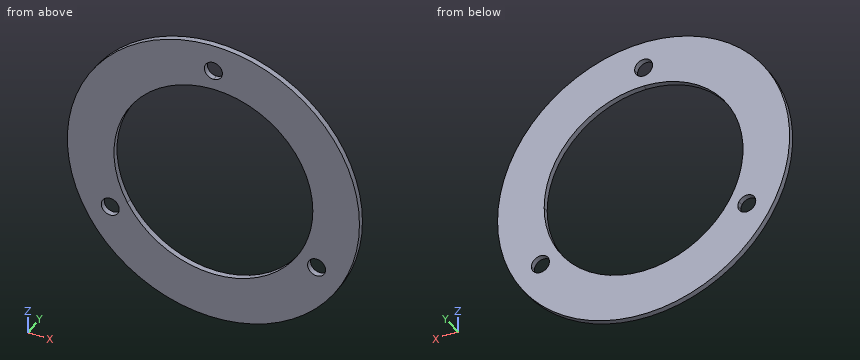
from build123d import *

# Parameters (mm, degrees)
F0_R     = 50.75
F1_DEPTH = 2


with BuildPart() as f1:
    # F0 (on Front) → F1 (new body)
    with BuildSketch(Plane.XZ):
        Circle(F0_R)
        with BuildLine():
            ThreePointArc((-32.725, -20.698007), (-38.868518, -21.506817), (-33.143671, -19.135507))
            ThreePointArc((-33.143671, -19.135507), (-32.831482, -19.889198), (-32.725, -20.698007))
        make_face(mode=Mode.SUBTRACT)
        with BuildLine():
            ThreePointArc((38.975, -20.698007), (35.04119, -23.716525), (33.143671, -19.135507))
            ThreePointArc((33.143671, -19.135507), (36.65881, -17.679489), (38.975, -20.698007))
        make_face(mode=Mode.SUBTRACT)
        with BuildLine():
            ThreePointArc((-29.921178, -17.275), (-29.921178, 17.275), (0, 34.55))
            ThreePointArc((0, 34.55), (24.430539, 24.430539), (34.55, 0))
            ThreePointArc((34.55, 0), (33.372737, -8.942198), (29.921178, -17.275))
            ThreePointArc((29.921178, -17.275), (0, -34.55), (-29.921178, -17.275))
        make_face(mode=Mode.SUBTRACT)
        with BuildLine():
            ThreePointArc((0, 38.271014), (-2.209709, 43.605723), (3.125, 41.396014))
            ThreePointArc((3.125, 41.396014), (2.209709, 39.186306), (0, 38.271014))
        make_face(mode=Mode.SUBTRACT)
    extrude(amount=F1_DEPTH)


solid = f1.part
The listing builds one solid part. Answer for the finished solid, in the listing's coordinates (mm). Give positions to 0.01 mm unless a question says otherwise; leave off trailing zeros. Write each loop counter-clockwise with the first axis right and the second up, starting at its lowest first coordinate (ties: lowest second). Pieces come first, ordered by that corner, then holes. Notation, with made-up numbers: (-25, -13.5) - (-1, -13.5) arc R9 ccw to (-1, -2.5) - close; hole circle Ø11 at (-26.5, 31). An arc over 180 degrees is marked (long way). One line per question, with ' | ' between items. Start each with the question number.
1. Section B-B, the plane y = -1.3 is taken. Count the separate pieces of the cut face and the enclosed holes in it, then the cut area to 3 significant figures.
2. Section C-C, the plane z = -2.5 is taken. Determine the outline of the cut face in (x, y), then the cut area to 3 significant figures.
3. Section A-A, the plane x = -35.85 is taken. Determine the outline of the cut face in (y, z).
4. Straight lines are drawn through the part: line 1 (X direction, y = -0.7, z = 41); line 2 (Z direction, x = -13.5, y = -0.3); line 3 (Z direction, x = 22, y = -0.4). For each, find the intervals that lie inside material, in ascending order.
5. Section D-D, the plane x = 43.5 is taken. Determine the outline of the cut face in (y, z).
Result:
1) separate pieces: 1 | enclosed holes: 4 | area: 4,250 mm2
2) outline: (-50.69, -2) - (-34.46, -2) - (-34.46, 0) - (-50.69, 0) - close; (34.46, -2) - (50.69, -2) - (50.69, 0) - (34.46, 0) - close | area: 64.9 mm2
3) outline: (-2, -35.92) - (0, -35.92) - (0, -23.82) - (-2, -23.82) - close; (-2, -17.57) - (0, -17.57) - (0, 35.92) - (-2, 35.92) - close
4) line 1: x = -29.91 to -3.1, 3.1 to 29.91 | line 2: z = -48.92 to -31.8, 31.8 to 48.92 | line 3: z = -45.73 to -26.64, 26.64 to 45.73
5) outline: (-2, -26.14) - (0, -26.14) - (0, 26.14) - (-2, 26.14) - close
